from build123d import *

# Parameters (mm, degrees)
SKETCH1_R                = 72.5
BOSS_EXTRUDE1_DEPTH      = 294
FILLET1_R                = 72.5
SKETCH2_R                = 63.5
BOSS_EXTRUDE2_DEPTH      = 431.8
SKETCH3_R                = 67
BOSS_EXTRUDE3_DEPTH      = 85.75
BOSS_EXTRUDE3_DEPTH_BACK = 78
CHAMFER1_SIZE            = 5
CHAMFER2_SIZE            = 16
CHAMFER2_SIZE2           = 7
SHELL1_T                 = -5


with BuildPart() as part:
    # Sketch1 → Boss-Extrude1 (new body)
    with BuildSketch(Plane.XY):
        Circle(SKETCH1_R)
    extrude(amount=BOSS_EXTRUDE1_DEPTH)

    # Fillet1
    fillet1_edges = [part.edges().sort_by_distance(p)[0] for p in [
        (-72.5, 0, 294),
    ]]
    fillet(fillet1_edges, radius=FILLET1_R)

    # Sketch2 → Boss-Extrude2 (add)
    with BuildSketch(Plane(origin=(0, 0, 0), x_dir=(1, 0, 0), z_dir=(0, 1, 0))):
        with Locations(Location((0, -85.5, 0), (0, 0, 270))):
            Circle(SKETCH2_R)
    extrude(amount=-BOSS_EXTRUDE2_DEPTH)

    # Sketch3 → Boss-Extrude3 (add, two sides)
    with BuildSketch(Plane.XY.offset(85.5)) as boss_extrude3_sk:
        with Locations((0, -431.8)):
            Circle(SKETCH3_R)
    extrude(amount=BOSS_EXTRUDE3_DEPTH)
    extrude(boss_extrude3_sk.sketch, amount=-BOSS_EXTRUDE3_DEPTH_BACK)

    # Chamfer1
    chamfer1_edges = [part.edges().sort_by_distance(p)[0] for p in [
        (-67, -431.8, 7.5),
    ]]
    chamfer(chamfer1_edges, length=CHAMFER1_SIZE)

    # Chamfer2
    chamfer2_edges = [part.edges().sort_by_distance(p)[0] for p in [
        (-67, -431.8, 171.25),
    ]]
    chamfer2_side = [part.faces().sort_by_distance(p)[0] for p in [
        (-67, -431.8, 91.875),
    ]]
    chamfer(chamfer2_edges, length=CHAMFER2_SIZE, length2=CHAMFER2_SIZE2, reference=chamfer2_side[0])

    # Shell1
    shell1_openings = [part.faces().sort_by_distance(p)[0] for p in [
        (0, -431.8, 171.25),
        (0, 0, 0),
    ]]
    offset(amount=SHELL1_T, openings=shell1_openings, kind=Kind.INTERSECTION)


solid = part.part
CAD build for the part. Positions are in the model's coordinates, mm. A direction names the side the tool comes from. Round coordinates to 2 decimals unless told otherwise and drop trailing zeros. Write each loop counter-clockwise with the first axis right and the second up, starting at its lowest first coordinate (ties: lowest second). Pieces come first, ordered by that corner, then holes.
(1) Slice it at B-B, the plane y = 0. Write the cut outline in (x, z).
(2) Mould opens along X. For faces 1 (the face through (-1, -431, 12.5)), 2 (the face through (-24.32, -220.08, 144.16)), 3 (the face through (13, -485, 171.25)) say: pulls with the +X half, pulls with the -X half, needs draft (parallel to the pull), parting line crosses it, or undercut.
(3) Drop flat-ended pins along their axis: P1, Ø2, axis at x = 33.5, y = -266, coming from the +Z side; P2, Ø10, axis at x = 47.5, y = -264, coming from the -Z side; P3, Ø3, axis at x = 14.5, z = 227.5, coming from the +Y side. Give the stop position or say it passes through.
(4) Slice it at A-A, the plane z = 85.5. Write the cut outline in (x, y).
(5) Slice it at D-D, the plane y = -174. Write the cut outline in (x, z), and give its area (3 significant figures).
(6) 3-axis set-ups, long thin cutter, end or side, ignore diameter. For faces 4 (the face through (-8.787, 66.926, 109.2)), 5 (the face through (-13.44, -492.326, 83.41)), 6 (the face through (48, -48, 0)), 7 (the face through (-7.855, -371.974, 170.473)), 8 (the face through (-1, -431, 7.5)): which of +Z, -Z, +X, -X, +Y, -Y reach the whole face in a straight line?
(7) Probe line 1 along Y through (x, z) = (-49.5, 17.5); line 2 along X through (y, z) = (-290.5, 85.5); line 3 along Z through (x, y) = (0, -300.5). List the from-to ranges inside material, lowest first.
From the geometry:
1. outline: (-72.5, 0) - (-67.5, 0) - (-67.5, 221.5) arc R67.5 cw to (67.5, 221.5) - (67.5, 0) - (72.5, 0) - (72.5, 221.5) arc R72.5 ccw to (-72.5, 221.5) - close
2. face 1: undercut
2. face 2: parting line crosses it
2. face 3: needs draft
3. P1: stops at z = 140.05
3. P2: stops at z = 38.32
3. P3: stops at y = 71.1
4. outline: (-63.5, -410.43) arc R67 ccw (long way) to (63.5, -410.43) - (63.5, -34.99) arc R72.5 ccw (long way) to (-63.5, -34.99) - close; hole (-58.5, -411.26) arc R62 ccw (long way) to (58.5, -411.26) - (58.5, -33.67) arc R67.5 ccw (long way) to (-58.5, -33.67) - close
5. outline: circle Ø127 at (0, 85.5); hole circle Ø117 at (0, 85.5)
5. area: 1,920 mm2
6. face 4: -Z
6. face 5: none
6. face 6: -Z, +X, -X, +Y, -Y
6. face 7: +Z
6. face 8: -Z, +X, -X, -Y
7. line 1: y = -476.95 to -469.13, -394.47 to -386.65, -52.97 to -45.89, 45.89 to 52.97
7. line 2: x = -63.5 to -58.5, 58.5 to 63.5
7. line 3: z = 22 to 27, 144 to 149
